Model file for the job. Use its own axes, mm. Face numbers are marked on the shaded views. Round coordinates to 2 decimals unless told otherwise and drop trailing zeros. Order: outer loops, then holes, each group sorted by start corner. A loop starts at its lowest first (then second) coordinate and runs counter-clockwise, first axis right, second up. Notation, with made-up numbers: (35.5, -35) -> (40.5, -35) arc R25 cw to (40.5, 1) -> close; hole circle Ø2 at (87, -6.75). An arc over 180 degrees is marked (long way). Answer as CSV lines item,"result".
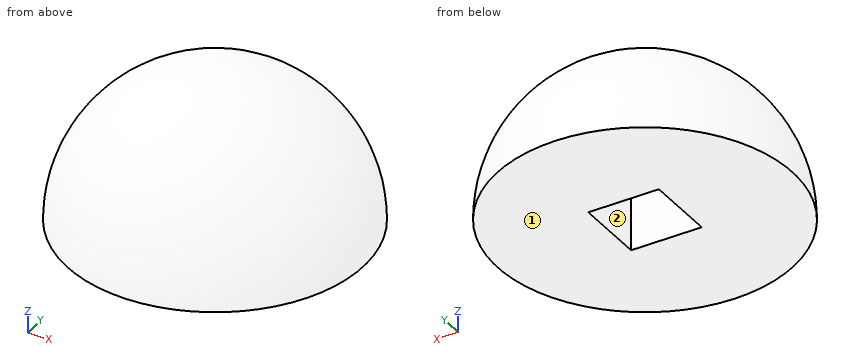
Autodesk Inventor part; units mm, degrees
ref_plane "YZ Plane" through (0, 0, 0) normal (1, 0, 0) x (0, 1, 0)
ref_plane "XZ Plane" through (0, 0, 0) normal (0, 1, 0) x (-1, 0, 0)
ref_plane "XY Plane" through (0, 0, 0) normal (0, 0, 1) x (1, 0, 0)
sketch "Sketch1" plane through (0, 0, 0) normal (0, 0, 1) x (1, 0, 0)
  circle A0 centre (0, 0) radius 6.35
  line L0 (0, 6.35) -> (0, -6.35)
  dimension "d0" = 12.7
revolve "Revolution1" add sketch "Sketch1" angle 180 about axis through (0, 6.35, 0) along (0, 1, 0) picked at (-3.484, 2.1167) contours L0 A0
sketch "Sketch3" plane through (0, 0, 0) normal (0, 0, -1) x (-1, 0, 0)
  line L0 (0, 0) -> (0, 1.524) construction
  line L1 (0, 1.524) -> (1.524, 1.524) construction
  line L2 (0, 0) -> (0, -1.524) construction
  line L3 (0, -1.524) -> (-1.524, -1.524) construction
  line L4 (1.524, 1.524) -> (-1.524, 1.524)
  line L5 (-1.524, 1.524) -> (-1.524, -1.524)
  line L6 (-1.524, -1.524) -> (1.524, -1.524)
  line L7 (1.524, -1.524) -> (1.524, 1.524)
  dimension "d5" = 1.524
  dimension "d11" = 1.524
  dimension "d12" = 1.524
  dimension "d13" = 1.524
extrude "Extrusion3" cut sketch "Sketch3" against normal blind 5.08
properties part number "ball"
Q1. Saw through at C-C (x = 0.75). Write the cut outline in (y, z), plus the area to 3 significant figures.
Checks:
outline,"(-6.31, 0) -> (-1.52, 0) -> (-1.52, 5.08) -> (1.52, 5.08) -> (1.52, 0) -> (6.31, 0) arc R6.31 ccw to start"
area,"47.0 mm²"
Q2. Saw through at B-B (z = 1.5). Write the cut outline in (x, y), plus the area to 3 significant figures.
Checks:
outline,"circle Ø12.34 at (0, 0); hole (-1.52, -1.52) -> (1.52, -1.52) -> (1.52, 1.52) -> (-1.52, 1.52) -> close"
area,"110 mm²"
Q3. Saw through at A-A (y = -0.5). Write the cut outline in (x, z).
Checks:
outline,"(-6.33, 0) -> (-1.52, 0) -> (-1.52, 5.08) -> (1.52, 5.08) -> (1.52, 0) -> (6.33, 0) arc R6.33 ccw to start"
Q4. Mould opens along Y. For the marked faces 1 and 2 say: +Y half, -Y half, draft (parallel to the pull), parting line (faces both ways), or undercut.
Checks:
face 1,"draft"
face 2,"undercut"
Q5. Flat gauge pins, fed straight in: pin 1 (3.5 mm diameter, centred on y = -0.5, z = 2, fed in from -X); pin 2 (3.5 mm diameter, centred on x = 0, y = 0.5, fed in from -Z); pin 3 (1.5 mm diameter, centred on y = 1, z = 5.5, fed in from +X); pin 4 (5 mm diameter, centred on x = 4, y = -0.5, fed in from +Z). Where does each tip first touch, or does it go through?
Checks:
pin 1,"x = -6.34"
pin 2,"z = 0"
pin 3,"x = 4.11"
pin 4,"z = 6.16"
Q6. Saw through at D-D (z = 5.5). Write the cut outline in (x, y).
Checks:
outline,"circle Ø6.35 at (0, 0)"
Q7. Wall check: L1, parallel to Y at x = 1, z = 1.5; L2, parallel to X at y = 0.5, z = 4.5; L3, parallel to Y at x = 0.5, z = 3.5. Give the ranges that are in metal, low to high. Write a range as [from, to].
Checks:
L1,"[-6.09, -1.52], [1.52, 6.09]"
L2,"[-4.45, -1.52], [1.52, 4.45]"
L3,"[-5.27, -1.52], [1.52, 5.27]"
